from build123d import *

# Parameters (mm, degrees)
SKETCH1_R           = 4
SKETCH1_R_2         = 2
SKETCH1_R_3         = 1.75
BOSS_EXTRUDE1_DEPTH = 3.175


with BuildPart() as part:
    # Sketch1 → Boss-Extrude1 (new body)
    with BuildSketch(Plane(origin=(0, 0, 0), x_dir=(0, 0, -1), z_dir=(1, 0, 0))):
        with BuildLine():
            Line((-240, -288), (-240, -310))
            ThreePointArc((-240, -310), (-242.928932188, -317.071067812), (-250, -320))
            Line((-250, -320), (-294, -320))
            ThreePointArc((-294, -320), (-301.071067812, -317.071067812), (-304, -310))
            Line((-304, -310), (-304, -288))
            Line((-304, -288), (-304, -59))
            ThreePointArc((-304, -59), (-282.033008589, -5.966991411), (-229, 16))
            Line((-229, 16), (-16, 16))
            Line((-16, 16), (10, 16))
            ThreePointArc((10, 16), (13.535533906, 14.535533906), (15, 11))
            Line((15, 11), (15, -11))
            ThreePointArc((15, -11), (13.535533906, -14.535533906), (10, -16))
            Line((10, -16), (-6.55, -16))
            ThreePointArc((-6.55, -16), (-18.252617229, -20.847382771), (-23.1, -32.55))
            Line((-23.1, -32.55), (-23.1, -201.8))
            ThreePointArc((-23.1, -201.8), (-26.028932188, -208.871067812), (-33.1, -211.8))
            Line((-33.1, -211.8), (-141.1, -211.8))
            ThreePointArc((-141.1, -211.8), (-148.171067812, -214.728932188), (-151.1, -221.8))
            Line((-151.1, -221.8), (-151.1, -252.6))
            ThreePointArc((-151.1, -252.6), (-154.028932188, -259.671067812), (-161.1, -262.6))
            Line((-161.1, -262.6), (-214.6, -262.6))
            ThreePointArc((-214.6, -262.6), (-232.560512242, -270.039487758), (-240, -288))
        make_face()
        with Locations((-256, -304)):
            Circle(SKETCH1_R, mode=Mode.SUBTRACT)
        Circle(SKETCH1_R, mode=Mode.SUBTRACT)
        with Locations((8, 0)):
            Circle(SKETCH1_R_2, mode=Mode.SUBTRACT)
        with Locations((0, -8)):
            Circle(SKETCH1_R_2, mode=Mode.SUBTRACT)
        with Locations((-8, 0)):
            Circle(SKETCH1_R_2, mode=Mode.SUBTRACT)
        with Locations((0, 8)):
            Circle(SKETCH1_R_2, mode=Mode.SUBTRACT)
        with Locations((-248, -304)):
            Circle(SKETCH1_R_2, mode=Mode.SUBTRACT)
        with Locations((-256, -312)):
            Circle(SKETCH1_R_2, mode=Mode.SUBTRACT)
        with Locations((-256, -296)):
            Circle(SKETCH1_R_2, mode=Mode.SUBTRACT)
        with Locations((-264, -304)):
            Circle(SKETCH1_R_2, mode=Mode.SUBTRACT)
        with Locations((-272, -304)):
            Circle(SKETCH1_R, mode=Mode.SUBTRACT)
        with Locations((-288, -312)):
            Circle(SKETCH1_R_2, mode=Mode.SUBTRACT)
        with Locations((-280, -304)):
            Circle(SKETCH1_R_2, mode=Mode.SUBTRACT)
        with Locations((-288, -296)):
            Circle(SKETCH1_R_2, mode=Mode.SUBTRACT)
        with Locations((-288, -304)):
            Circle(SKETCH1_R, mode=Mode.SUBTRACT)
        with Locations((-296, -304)):
            Circle(SKETCH1_R_2, mode=Mode.SUBTRACT)
        with Locations((-171.05, -252.6)):
            Circle(SKETCH1_R_2, mode=Mode.SUBTRACT)
        with Locations((-179.05, -244.6)):
            Circle(SKETCH1_R_2, mode=Mode.SUBTRACT)
        with Locations((-171.05, -236.6)):
            Circle(SKETCH1_R_2, mode=Mode.SUBTRACT)
        with Locations((-163.05, -244.6)):
            Circle(SKETCH1_R_2, mode=Mode.SUBTRACT)
        with Locations((-179.05, -228.6)):
            Circle(SKETCH1_R_2, mode=Mode.SUBTRACT)
        with Locations((-171.05, -220.6)):
            Circle(SKETCH1_R_2, mode=Mode.SUBTRACT)
        with Locations((-163.05, -228.6)):
            Circle(SKETCH1_R_2, mode=Mode.SUBTRACT)
        with Locations((-179.05, -212.6)):
            Circle(SKETCH1_R_2, mode=Mode.SUBTRACT)
        with Locations((-171.05, -204.6)):
            Circle(SKETCH1_R_2, mode=Mode.SUBTRACT)
        with Locations((-163.05, -212.6)):
            Circle(SKETCH1_R_2, mode=Mode.SUBTRACT)
        with Locations((-179.05, -196.6)):
            Circle(SKETCH1_R_2, mode=Mode.SUBTRACT)
        with Locations((-171.05, -188.6)):
            Circle(SKETCH1_R_2, mode=Mode.SUBTRACT)
        with Locations((-163.05, -196.6)):
            Circle(SKETCH1_R_2, mode=Mode.SUBTRACT)
        with Locations((-179.05, -180.6)):
            Circle(SKETCH1_R_2, mode=Mode.SUBTRACT)
        with Locations((-171.05, -172.6)):
            Circle(SKETCH1_R_2, mode=Mode.SUBTRACT)
        with Locations((-163.05, -180.6)):
            Circle(SKETCH1_R_2, mode=Mode.SUBTRACT)
        with Locations((-179.05, -164.6)):
            Circle(SKETCH1_R_2, mode=Mode.SUBTRACT)
        with Locations((-171.05, -156.6)):
            Circle(SKETCH1_R_2, mode=Mode.SUBTRACT)
        with Locations((-163.05, -164.6)):
            Circle(SKETCH1_R_2, mode=Mode.SUBTRACT)
        with Locations((-179.05, -148.6)):
            Circle(SKETCH1_R_2, mode=Mode.SUBTRACT)
        with Locations((-171.05, -140.6)):
            Circle(SKETCH1_R_2, mode=Mode.SUBTRACT)
        with Locations((-163.05, -148.6)):
            Circle(SKETCH1_R_2, mode=Mode.SUBTRACT)
        with Locations((-179.05, -132.6)):
            Circle(SKETCH1_R_2, mode=Mode.SUBTRACT)
        with Locations((-171.05, -124.6)):
            Circle(SKETCH1_R_2, mode=Mode.SUBTRACT)
        with Locations((-163.05, -132.6)):
            Circle(SKETCH1_R_2, mode=Mode.SUBTRACT)
        with Locations((-179.05, -116.6)):
            Circle(SKETCH1_R_2, mode=Mode.SUBTRACT)
        with Locations((-171.05, -108.6)):
            Circle(SKETCH1_R_2, mode=Mode.SUBTRACT)
        with Locations((-163.05, -116.6)):
            Circle(SKETCH1_R_2, mode=Mode.SUBTRACT)
        with Locations((-286.5, -117.1)):
            Circle(SKETCH1_R_3, mode=Mode.SUBTRACT)
        with Locations((-198.5, -117.1)):
            Circle(SKETCH1_R_3, mode=Mode.SUBTRACT)
        with Locations((-198.5, -245.1)):
            Circle(SKETCH1_R_3, mode=Mode.SUBTRACT)
        with Locations((-286.5, -245.1)):
            Circle(SKETCH1_R_3, mode=Mode.SUBTRACT)
        with Locations((-133.6, -61.3)):
            Circle(SKETCH1_R_3, mode=Mode.SUBTRACT)
        with Locations((-45.6, -61.3)):
            Circle(SKETCH1_R_3, mode=Mode.SUBTRACT)
        with Locations((-45.6, -189.3)):
            Circle(SKETCH1_R_3, mode=Mode.SUBTRACT)
        with Locations((-133.6, -189.3)):
            Circle(SKETCH1_R_3, mode=Mode.SUBTRACT)
    extrude(amount=-BOSS_EXTRUDE1_DEPTH)


solid = part.part
CAD build for the part. Positions are in the model's coordinates, mm. Coordinates: 2 decimals unless noted, no trailing zeros. Order: outer loops, then holes, each group sorted by start corner. A loop starts at its lowest first (then second) coordinate and runs counter-clockwise, first axis right, second up. Notation, with made-up numbers: (28, -20) -> (69, -20) arc R23 ccw to (69, 9) -> close; hole circle Ø9 at (-37, -11). An arc over 180 degrees is marked (long way). Answer in a Markdown table with one row per item.
1) Drill centre lines: line 1 (Z direction, x = -2.2, y = -117.1); line 2 (Y direction, x = -1.7, z = 50); line 3 (Z direction, x = -2.3, y = -177). Where is each one in solid material? Low to high.
Check values:
| item | result |
|---|---|
| line 1 | 23.1 to 161.11, 164.99 to 177.11, 180.99 to 196.75, 200.25 to 284.75, 288.25 to 304 |
| line 2 | -211.8 to 16 |
| line 3 | 23.1 to 304 |
2) Band-saw the part on C-C (z = 74). List the corners of the cut face in (x, y) (3 decimals), and give its area (3 significant figures).
Check values:
| item | result |
|---|---|
| outline | (-3.175, -211.8) -> (0, -211.8) -> (0, 16) -> (-3.175, 16) -> close |
| area | 723 mm2 |
3) Band-saw the part on A-A (z = 272). List the corners of the cut face in (x, y) (3 decimals), and give its area (3 significant figures).
Check values:
| item | result |
|---|---|
| outline | (-3.175, -320) -> (0, -320) -> (0, -308) -> (-3.175, -308) -> close; (-3.175, -300) -> (0, -300) -> (0, 2.449) -> (-3.175, 2.449) -> close |
| area | 998 mm2 |
4) Band-saw the part on D-D (z = 191). List the corners of the cut face in (x, y) (3 decimals), and give its area (3 significant figures).
Check values:
| item | result |
|---|---|
| outline | (-3.175, -262.6) -> (0, -262.6) -> (0, 16) -> (-3.175, 16) -> close |
| area | 885 mm2 |
5) Band-saw the part on B-B (x = -0.9). Give the number of separate pieces and of enclosed holes in the cut face, and give its area (3 significant figures).
Check values:
| item | result |
|---|---|
| separate pieces | 1 |
| enclosed holes | 52 |
| area | 74,800 mm2 |
6) Flat gauge pins, fed straight in: P1, Ø1.6, axis at x = -1, z = 191.5, coming from the -Y side; P2, Ø1, axis at x = -1.5, y = -27, coming from the +Z side; P3, Ø1.6, axis at x = -2, y = -153, coming from the -Z side. Where does each tip first touch, or does it go through?
Check values:
| item | result |
|---|---|
| P1 | y = -262.6 |
| P2 | z = 297.06 |
| P3 | z = 23.1 |
7) Mould opens along Z. For faces 1 (the face through (-1.565, -20.719, 18.123)), 2 (the face through (-1.6, -306.4, 275.2)), 3 (the face through (-1.57, -317.15, 300.99)) say: pulls with the +Z half, pulls with the -Z half, needs draft (parallel to the pull), parting line crosses it, or undercut.
Check values:
| item | result |
|---|---|
| face 1 | pulls with the -Z half |
| face 2 | undercut |
| face 3 | pulls with the +Z half |
